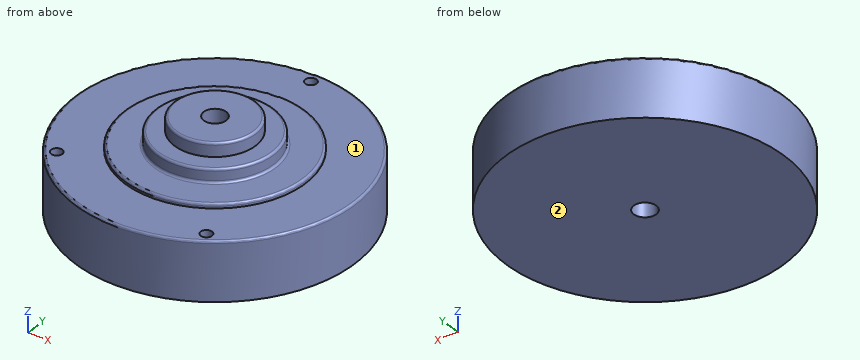
```python
from build123d import *

# Parameters (mm, degrees)
ESQUISSE2_R             = 2.5
ENL_V_MAT_EXTRU_1_DEPTH = 49.187135213
CONG_1_R                = 0.5
ESQUISSE3_R             = 1.25
ENL_V_MAT_EXTRU_2_DEPTH = 5


with BuildPart() as part:
    # Esquisse1 → Révolution1 (revolve)
    with BuildSketch(Plane(origin=(0, 0, 0), x_dir=(1, 0, 0), z_dir=(0, 1, 0)), mode=Mode.PRIVATE) as r_volution1_sk:
        Polygon((0, 0), (31, 0), (31, -13), (20, -13), (20, -14), (13, -14), (13, -17), (9, -17), (9, -20), (0, -20), align=None)
    revolve(r_volution1_sk.sketch.rotate(Axis((0, 0, 0), (0, 0, 1)), 180), axis=Axis((0, 0, 0), (0, 0, 1)))

    # Esquisse2 → Enlèv. mat.-Extru.1 (cut, through all)
    with BuildSketch(Plane.XY.offset(20)):
        Circle(ESQUISSE2_R)
    extrude(amount=-ENL_V_MAT_EXTRU_1_DEPTH, mode=Mode.SUBTRACT)

    # Congé1
    cong_1_edges = [part.edges().sort_by_distance(p)[0] for p in [
        (9, 0, 20),
        (13, 0, 17),
        (13, 0, 14),
        (20, 0, 14),
        (31, 0, 13),
    ]]
    fillet(cong_1_edges, radius=CONG_1_R)

    # Esquisse3 → Enlèv. mat.-Extru.2 (cut)
    with BuildSketch(Plane.XY.offset(13)):
        with Locations((0, 28.5)):
            Circle(ESQUISSE3_R)
        with Locations((-22.07133422, -18.030701754)):
            Circle(ESQUISSE3_R)
        with Locations((16.028756412, -23.565418899)):
            Circle(ESQUISSE3_R)
    extrude(amount=-ENL_V_MAT_EXTRU_2_DEPTH, mode=Mode.SUBTRACT)


solid = part.part
```
Here's how the part is built. I have some questions about the finished solid (model axes, mm). Face numbers are marked on the shaded views. A direction names the side the tool comes from. Give positions to 0.01 mm unless a question says otherwise; leave off trailing zeros. Write each loop counter-clockwise with the first axis right and the second up, starting at its lowest first coordinate (ties: lowest second). Pieces come first, ordered by that corner, then holes. Notation, with made-up numbers: (29, 9) -> (40, 9) arc R17 cw to (40, 23) -> close; hole circle Ø4 at (15, 60.25). An arc over 180 degrees is marked (long way). Write each question's results on one line, items separated by ' | '.
Item 1: Suppose I cut it at D-D on z = 18.5. Write out the boundary of the cut face in (x, y).
Output:
outline: circle Ø18 at (0, 0); hole circle Ø5 at (0, 0)
Item 2: For pin 1 Ø8 at (y, z) = (-13, 6) entering from +X; pin 2 Ø3 at (x, y) = (-22, -18.5) entering from +Z; pin 3 Ø2 at (x, z) = (2, 11.5) entering from -Y, each with a flat end and sliding along its axis, tell me the tip position at first contact or that it passes through.
Output:
pin 1: stops at x = 29.66 | pin 2: stops at z = 13 | pin 3: stops at y = -30.98
Item 3: If I drill on L1, parallel to Y at x = 0, z = 9.55; L2, parallel to Y at x = 0, z = 7.75; L3, parallel to Y at x = 1, z = 10.5, over which ranges is the centre line in solid material (lowest first)?
Output:
L1: y = -31 to -2.5, 2.5 to 27.25, 29.75 to 31 | L2: y = -31 to -2.5, 2.5 to 31 | L3: y = -30.98 to -2.29, 2.29 to 27.75, 29.25 to 30.98
Item 4: On a 3-axis mill with a long thin cutter (end or side, diameter ignored), from which of +Z, -Z, +X, -X, +Y, -Y can I reach the whole of each face in a straight line? I mean the marked faces 1 and 2. Say none if no direction works.
Output:
face 1: +Z | face 2: -Z, +X, -X, +Y, -Y
Item 5: Suppose I cut it at C-C on z = 15.25. Write out the boundary of the cut face in (x, y), plus the area to 3 significant figures.
Output:
outline: circle Ø26 at (0, 0); hole circle Ø5 at (0, 0) | area: 511 mm^2
